Work out the finished part from the listing and answer in its coordinate system (mm). Face numbers are marked on the shaded views. A direction names the side the tool comes from. Coordinates: 2 decimals unless noted, no trailing zeros. Loops run counter-clockwise (first coordinate to the right, second up) from the corner with the lowest first, then second, coordinate; pieces in that order, holes last. Notation, with made-up numbers: (-26, 86) -> (-19, 86) arc R28 cw to (-19, 111) -> close; hole circle Ø9 at (24, 89.5). An arc over 180 degrees is marked (long way). Use a Markdown table: item, result.
from build123d import *

# Parameters (mm, degrees)
F0_W     = 113
F0_H     = 32
F1_DEPTH = 64
F2_W     = 25
F2_H     = 51
F2_H_2   = 34
F2_W_2   = 35
F2_H_3   = 17
F3_DEPTH = 32.001
F5_R     = 5.5
F4_R     = 5.5
F7_DEPTH = 25
F8_DEPTH = 88.001


with BuildPart() as f1:
    # F0 (on Top) → F1 (new body)
    with BuildSketch(Plane.XY):
        with Locations((13.7222270072, 16)):
            Rectangle(F0_W, F0_H)
    extrude(amount=F1_DEPTH)

    # F2 (on face) → F3 (cut, through all)
    with BuildSketch(Plane.XZ):
        with Locations((-30.2777729928, 38.5)):
            Rectangle(F2_W, F2_H)
        with Locations((13.7222270072, 47)):
            Rectangle(F2_W, F2_H_2)
        with Locations((13.7222270072, 8.5)):
            Rectangle(F2_W_2, F2_H_3)
        with Locations((57.7222270072, 38.5)):
            Rectangle(F2_W, F2_H)
    extrude(amount=-F3_DEPTH, mode=Mode.SUBTRACT)

    # F5 (on face) + F4 (on face) → F7 (cut)
    with BuildSketch(Plane.XY.offset(13)):
        with Locations((57.7222270072, 16)):
            Circle(F5_R)
        Polygon((60.2222270072, 0), (70.2222270072, 0), (70.2222270072, 10), align=None)
    with BuildSketch(Plane.XY.offset(13)):
        with Locations((-30.2777729928, 16)):
            Circle(F4_R)
        Polygon((-42.7777729928, 10), (-42.7777729928, 0), (-32.7777729928, 0), align=None)
    extrude(amount=-F7_DEPTH, mode=Mode.SUBTRACT)

    # F6 (on face) → F8 (cut, through all)
    with BuildSketch(Plane.YZ.offset(45.2222270072)):
        with BuildLine():
            Line((9.8946494696, 48.2304024078), (15.3522470821, 39.5323562129))
            ThreePointArc((15.3522470821, 39.5323562129), (15.6757197327, 39.5080940928), (16, 39.5))
            ThreePointArc((16, 39.5), (16.3242802673, 39.5080940928), (16.6477529179, 39.5323562129))
            Line((16.6477529179, 39.5323562129), (22.1053505304, 48.2304024078))
            ThreePointArc((22.1053505304, 48.2304024078), (16, 52.5), (9.8946494696, 48.2304024078))
        make_face()
        with BuildLine():
            ThreePointArc((9.8946494696, 48.2304024078), (10.4940846857, 42.5453080381), (15.3522470821, 39.5323562129))
            Line((15.3522470821, 39.5323562129), (9.8946494696, 48.2304024078))
        make_face()
        with BuildLine():
            Line((22.1053505304, 48.2304024078), (16.6477529179, 39.5323562129))
            ThreePointArc((16.6477529179, 39.5323562129), (20.8197714659, 41.6388300862), (22.5, 46))
            ThreePointArc((22.5, 46), (22.4005772571, 47.1325240731), (22.1053505304, 48.2304024078))
        make_face()
    extrude(amount=-F8_DEPTH, mode=Mode.SUBTRACT)


solid = f1.part
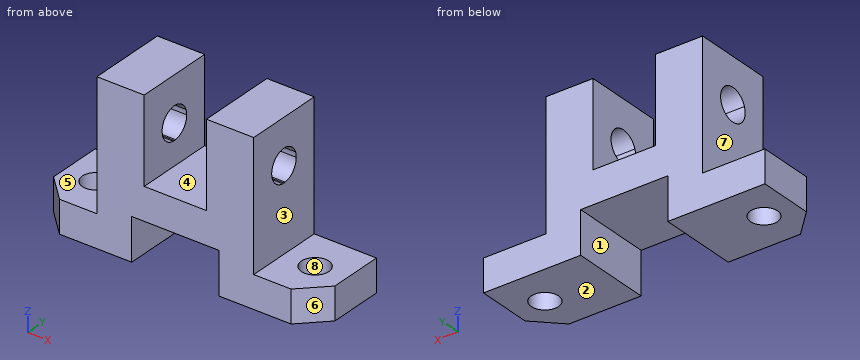
Q1. Section B-B on x = -12 is taken. Determine the outline of the cut face in (y, z), and give its area (3 significant figures).
Solved:
| item | result |
|---|---|
| outline | (0, 0) -> (32, 0) -> (32, 64) -> (0, 64) -> close; hole circle Ø13 at (16, 46) |
| area | 1,920 mm² |
Q2. Determine the mould class of the marked faces 6, 7 and 8 for opening direction X: pulls with the +X half, pulls with the -X half, needs draft (parallel to the pull), parting line crosses it, or undercut.
Solved:
| item | result |
|---|---|
| face 6 | pulls with the +X half |
| face 7 | pulls with the -X half |
| face 8 | undercut |
Q3. Consider line 1 (X direction, y = 26, z = 36); line 2 (Y direction, x = -12, z = 49.5); line 3 (X direction, y = 28.5, z = 12.5). Determine where each line is inside the solid, lowest interval first. Write a range as [from, to].
Solved:
| item | result |
|---|---|
| line 1 | [-17.78, 1.22], [26.22, 45.22] |
| line 2 | [0, 10.52], [21.48, 32] |
| line 3 | [-42.78, -3.78], [31.22, 70.22] |
Q4. Section D-D on z = 26.5 is taken. Determine the outline of the cut face in (x, y), and give its area (3 significant figures).
Solved:
| item | result |
|---|---|
| outline | (-17.78, 0) -> (45.22, 0) -> (45.22, 32) -> (-17.78, 32) -> close |
| area | 2,020 mm² |
Q5. For the marked faces 1, 2, 3, 4 and 5, determine the directions among +Z, -Z, +X, -X, +Y, -Y from which every point of the face is accessible in a straight line to the end or side of a thin tool.
Solved:
| item | result |
|---|---|
| face 1 | -Z, +Y, -Y |
| face 2 | -Z, +X, -X, +Y, -Y |
| face 3 | +Z, +X, +Y, -Y |
| face 4 | +Z, +Y, -Y |
| face 5 | +Z, -X, +Y, -Y |
Q6. Given pin 1 Ø10 at (x, y) = (25.5, 27.5) entering from -Z; pin 2 Ø9.5 at (y, z) = (23.5, 43) entering from +X; pin 3 Ø4 at (y, z) = (20.5, 49.5) entering from -X, each flat-ended and moving along its own axis, determine where each tip first touches the part or whether it passes through.
Solved:
| item | result |
|---|---|
| pin 1 | z = 17 |
| pin 2 | x = 45.22 |
| pin 3 | x = -17.78 |
Q7. Section C-C on y = 12 is taken. State how many separate pieces and enclosed holes the cut face has, and give its area (3 significant figures).
Solved:
| item | result |
|---|---|
| separate pieces | 5 |
| enclosed holes | 0 |
| area | 2,650 mm² |
Q8. Section A-A on z = 56 is taken. Determine the outline of the cut face in (x, y).
Solved:
| item | result |
|---|---|
| outline | (-17.78, 0) -> (1.22, 0) -> (1.22, 32) -> (-17.78, 32) -> close; (26.22, 0) -> (45.22, 0) -> (45.22, 32) -> (26.22, 32) -> close |
